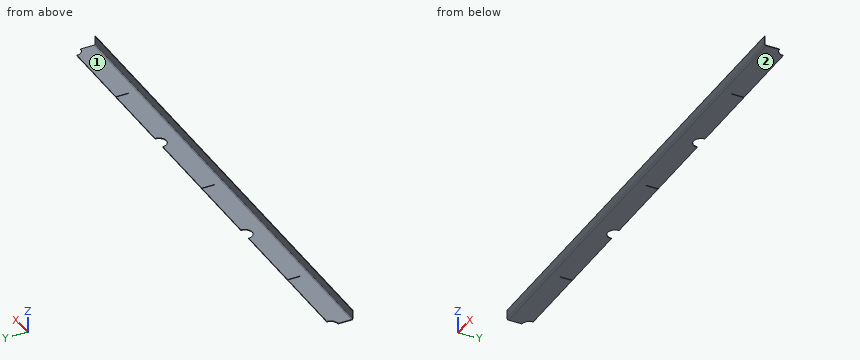
Autodesk Inventor part; units mm, degrees
ref_plane "YZ Plane" through (0, 0, 0) normal (1, 0, 0) x (0, 1, 0)
ref_plane "XZ Plane" through (0, 0, 0) normal (0, 1, 0) x (-1, 0, 0)
ref_plane "XY Plane" through (0, 0, 0) normal (0, 0, 1) x (1, 0, 0)
sketch "Sketch1" plane through (0, 0, 0) normal (0, 0, 1) x (1, 0, 0)
  line L0 (-750, 67.6691) -> (750, 67.6691)
  line L1 (750, 67.6691) -> (750, 0)
  line L2 (750, 0) -> (-750, 0)
  line L3 (-750, 0) -> (-750, 67.6691)
  point P0 (0, 0)
  point P1 (0, 0)
  dimension "d0" = 1500
  dimension "d1" = 67.669
extrude "Plate1" add sketch "Sketch1" along normal blind 2
sketch "Sketch2" plane through (750, 2, 0) normal (0, -1, 0) x (1, 0, 0)
  line L0 (-1500, 0) -> (0, 0)
  line L1 (0, 0) -> (0, 30)
  line L2 (0, 30) -> (-1500, 30)
  line L3 (-1500, 30) -> (-1500, 0)
edge flange "Flange1" height 30 angle 90 thickness 2 bend radius 2.75 thickness toward (0, -1, 0) relief round relief width 2 relief depth 1 edges at (0, 0, 2) wall of the first edge with corners at (-750, 2, 0) (750, 2, 0) (750, 2, 30) (-750, 2, 30)
bend "Bend1"
corner "Corner1"
sketch "Sketch5" plane through (0, 0, 0) normal (0, 0, -1) x (-1, 0, 0)
  line L0 (750, 67.6691) -> (-750, 67.6691)
  line L1 (-1, 30) -> (-1, 67.6691)
  line L2 (750, 0) -> (-750, 0)
  line L3 (-1, 30) -> (1, 30)
  line L4 (1, 30) -> (1, 67.6691)
  point P0 (0, 0)
  point P1 (0, 30)
  point P2 (0, 0)
  dimension "d27" = 2
  dimension "d29" = 30
extrude "Extrusion1" cut sketch "Sketch5" against normal through all
pattern_linear "Rectangular Pattern1" count 3 spacing 500 along (1, 0, 0) of "Extrusion1" first direction both ways yes
sketch "Sketch6" plane through (0, 0, 0) normal (0, 0, -1) x (-1, 0, 0)
  line L0 (-750, 67.6691) -> (-750, 4.75)
  circle A0 centre (-750, 67.6691) radius 22.5
  line L1 (-750, 67.6691) -> (750, 67.6691)
  line L2 (-1, 67.6691) -> (-1, 30)
  line L3 (-499, 30) -> (-499, 67.6691)
  line L4 (-1, 30) -> (-499, 30) construction
  circle A1 centre (-250, 67.6691) radius 22.5
  point P0 (0, 0)
  point P1 (-727.5, 67.6691)
  point P2 (-750, 45.1691)
  point P3 (-250, 30)
  dimension "d24" = 45
extrude "Extrusion2" cut sketch "Sketch6" along normal mid plane 30 contours L1 A0 L0 | A1 L1 | L1 A1 picked at (-748.3311, 52.8571)
mirror "Mirror1" about plane through (0, 0, 0) normal (1, 0, 0) of "Extrusion2"
sketch "Sketch7" plane through (0, 0, 2) normal (0, 0, 1) x (1, 0, 0)
  arc A0 (-750, 45.1691) -> (-727.5, 67.6691) centre (-750, 67.6691) ccw
  line L0 (-750, 4.75) -> (-750, 45.1691)
  line L1 (-750, 4.75) -> (750, 4.75)
  line L2 (750, 45.1691) -> (750, 4.75)
  arc A1 (727.5, 67.6691) -> (750, 45.1691) centre (750, 67.6691) ccw
  line L3 (501, 67.6691) -> (727.5, 67.6691)
  line L4 (501, 67.6691) -> (501, 30)
  line L5 (501, 30) -> (499, 30)
  line L6 (499, 30) -> (499, 67.6691)
  line L7 (1, 67.6691) -> (227.5, 67.6691)
  line L8 (1, 67.6691) -> (1, 30)
  line L9 (1, 30) -> (-1, 30)
  line L10 (-1, 30) -> (-1, 67.6691)
  line L11 (-499, 67.6691) -> (-272.5, 67.6691)
  line L12 (-499, 67.6691) -> (-499, 30)
  line L13 (-499, 30) -> (-501, 30)
  line L14 (-501, 30) -> (-501, 67.6691)
  line L15 (-727.5, 67.6691) -> (-501, 67.6691)
  line L16 (649, 32.2095) -> (651, 32.2095)
  line L17 (651, 32.2095) -> (651, 40.2095)
  line L18 (651, 40.2095) -> (649, 40.2095)
  line L19 (649, 40.2095) -> (649, 32.2095)
  line L20 (-750, 4.75) -> (750, 4.75)
  line L21 (650, 4.75) -> (650, 67.6691) construction
  line L22 (637, 32.2095) -> (639, 32.2095)
  line L23 (639, 32.2095) -> (639, 40.2095)
  line L24 (639, 40.2095) -> (637, 40.2095)
  line L25 (637, 40.2095) -> (637, 32.2095)
  line L26 (272.5, 67.6691) -> (499, 67.6691)
  arc A2 (227.5, 67.6691) -> (272.5, 67.6691) centre (250, 67.6691) ccw
  line L27 (-227.5, 67.6691) -> (-1, 67.6691)
  arc A3 (-272.5, 67.6691) -> (-227.5, 67.6691) centre (-250, 67.6691) ccw
  point P0 (0, 0)
  point P1 (650, 32.2095)
  point P2 (649, 36.2095)
  point P3 (650, 36.2095)
  point P4 (639, 36.2095)
  dimension "d30" = 2
  dimension "d31" = 8
  dimension "d32" = 100
  dimension "d33" = 2
  dimension "d34" = 8
  dimension "d35" = 10
extrude "Extrusion3" [suppressed]
mirror "Mirror2" [suppressed]
sketch "Sketch9" plane through (0, 0, 2) normal (0, 0, 1) x (1, 0, 0)
  line L0 (494, 62.6691) -> (494, 50.6691) construction
  line L1 (494, 50.6691) -> (294, 50.6691) construction
  line L2 (294, 50.6691) -> (294, 62.6691) construction
  line L3 (294, 62.6691) -> (494, 62.6691) construction
  line L4 (499, 30) -> (499, 67.6691)
  line L5 (1, 67.6691) -> (499, 67.6691)
  point P0 (0, 0)
  dimension "d40" = 200
  dimension "d41" = 12
  dimension "d42" = 5
  dimension "d43" = 5
mark "Mark2"
equation "\"d1\" = Стрингер_2"
equation "\"d27\" = d18"
equation "\"d29\" = Стрингер_глубина_паза"
equation "\"d43\" = d42"
equation "\"d2\" = Thickness"
equation "\"d3\" = BendReliefWidth"
equation "\"d4\" = BendReliefDepth"
equation "\"d5\" = MinimumRemnant"
equation "\"d6\" = TransitionRadius"
equation "\"d9\" = BendRadius"
equation "\"d10\" = CornerReliefSize"
equation "\"d11\" = GapSize"
equation "\"d12\" = JacobiRadiusSize"
equation "\"BendReliefWidth\" = Thickness"
equation "\"BendReliefDepth\" = 0.5 * Thickness"
equation "\"CornerReliefSize\" = 4 * Thickness"
equation "\"MinimumRemnant\" = 2 * Thickness"
equation "\"TransitionRadius\" = BendRadius"
equation "\"JacobiRadiusSize\" = BendRadius"
equation "\"GapSize\" = Thickness"
equation "\"d18\" = Thickness"
equation "\"qqqqqq\" = 67.35706"
properties part number "МОО 062 stringer спина ^^" material "Stainless Steel"
Input: part model. Units: mm. Frame: model coordinates. Face numbers are marked on the shaded views. A direction names the side the tool comes from. Give positions to 0.01 mm unless a question says otherwise; leave off trailing zeros. Order: outer loops, then holes, each group sorted by start corner. A loop starts at its lowest first (then second) coordinate and runs counter-clockwise, first axis right, second up. Notation, with made-up numbers: (-1.75, -29.5) - (43.25, -29.5) arc R28 ccw to (43.25, 5.5) - close; hole circle Ø2 at (19.25, 49.5). An arc over 180 degrees is marked (long way). Use a Markdown table: item, result.
(1) Pin query (flat end, axial travel): pin 1 (1 mm diameter, centred on x = 500, z = 0.5, fed in from +Y); pin 2 (3 mm diameter, centred on x = -60, z = 17, fed in from +Y); pin 3 (0.6 mm diameter, centred on y = 54, z = 1, fed in from -X). Return the tip coordinate at first contact, or that it passes through.
Computed values:
| item | result |
|---|---|
| pin 1 | stops at y = 30 |
| pin 2 | stops at y = 2 |
| pin 3 | stops at x = -732.36 |
(2) Access query for the marked faces 1 and 2. Directions: +Z, -Z, +X, -X, +Y, -Y. A direction counts if a zero-diameter tool reaches every point of the face in a straight line with its end or side. Return the directions, or none.
Computed values:
| item | result |
|---|---|
| face 1 | +Z, +X, -X, +Y |
| face 2 | -Z, +X, -X, +Y, -Y |
(3) Section query C-C (z = 13.25). Output: boundary loops of the cut face in (x, y), then the cut area to 3 significant figures.
Computed values:
| item | result |
|---|---|
| outline | (-750, 0) - (750, 0) - (750, 2) - (-750, 2) - close |
| area | 3,000 mm2 |
(4) Section query A-A (x = 250). Output: boundary loops of the cut face in (y, z), then the cut area to 3 significant figures.
Computed values:
| item | result |
|---|---|
| outline | (0, 4.75) arc R4.75 ccw to (4.75, 0) - (45.17, 0) - (45.17, 2) - (4.75, 2) arc R2.75 cw to (2, 4.75) - (2, 30) - (0, 30) - close |
| area | 143 mm2 |
(5) Line query: line 1 (Y direction, x = 187.5, z = 27.25); line 2 (Y direction, x = 377.5, z = 1.5). Output: solid intervals per line, ascending. Write a range as from..to.
Computed values:
| item | result |
|---|---|
| line 1 | y = 0..2 |
| line 2 | y = 1.29..67.67 |
(6) Section query B-B (x = 402.5). Output: boundary loops of the cut face in (y, z), then the cut area to 3 significant figures.
Computed values:
| item | result |
|---|---|
| outline | (0, 4.75) arc R4.75 ccw to (4.75, 0) - (67.67, 0) - (67.67, 2) - (4.75, 2) arc R2.75 cw to (2, 4.75) - (2, 30) - (0, 30) - close |
| area | 188 mm2 |
